Input: dimensioned drawing with shaded views. Units: mm. Origin: part minimum x, y, z. A direction names the side the tool comes from. Round coordinates to 2 decimals unless told otherwise and drop trailing zeros. Order: outer loops, then holes, each group sorted by start corner. A loop starts at its lowest first (then second) coordinate and runs counter-clockwise, first axis right, second up. Notation, with made-up numbers: M -25,43.5 L 30,43.5 A21 cw 30,63.5 Z; hole C 22.5,66.25 d6. An arc over 180 degrees is marked long. Use one line per item in the form item = value. Start each with the question number.
Q1. Section D-D (x = 43). Return the cut outline in (y, z).
Q2. Material intervals for probe 1 along Y at (x, z) = (40, 2.5); probe 2 along Z at (x, y) = (7, 20.5); probe 3 along X at (y, z) = (29.5, 37.5), sorted ascending.
Q3. Pull-direction query (Z, two-part tool) for the marked faces 3, 4 and 5; classes: pulls with the +Z half, pulls with the -Z half, needs draft (parallel to the pull), parting line crosses it, or undercut.
Q4. Contact query for flat-ended pins moving along their axis: pin 1 (1.5 mm diameter, centred on y = 18, z = 12.5, fed in from -X); pin 2 (5 mm diameter, centred on x = 14, y = 3.5, fed in from +Z); pin 3 (16 mm diameter, centred on y = 21, z = 30, fed in from +X); pin 4 (20 mm diameter, centred on x = 31, y = 12, fed in from +Z). Output: stop coordinate, or through.
Q5. Section B-B (x = 7.5). Return the cut outline in (y, z).
Q6. Section A-A (z = 28). Return the cut outline in (x, y).
Q7. Section C-C (y = 29). Return the cut outline in (x, z), plus the area to 3 significant figures.
Q8. Reachability of the marked faces 1 and 2 from +Z, -Z, +X, -X, +Y, -Y: full face, straight path, thin tool, end or side. Return the list, or none.
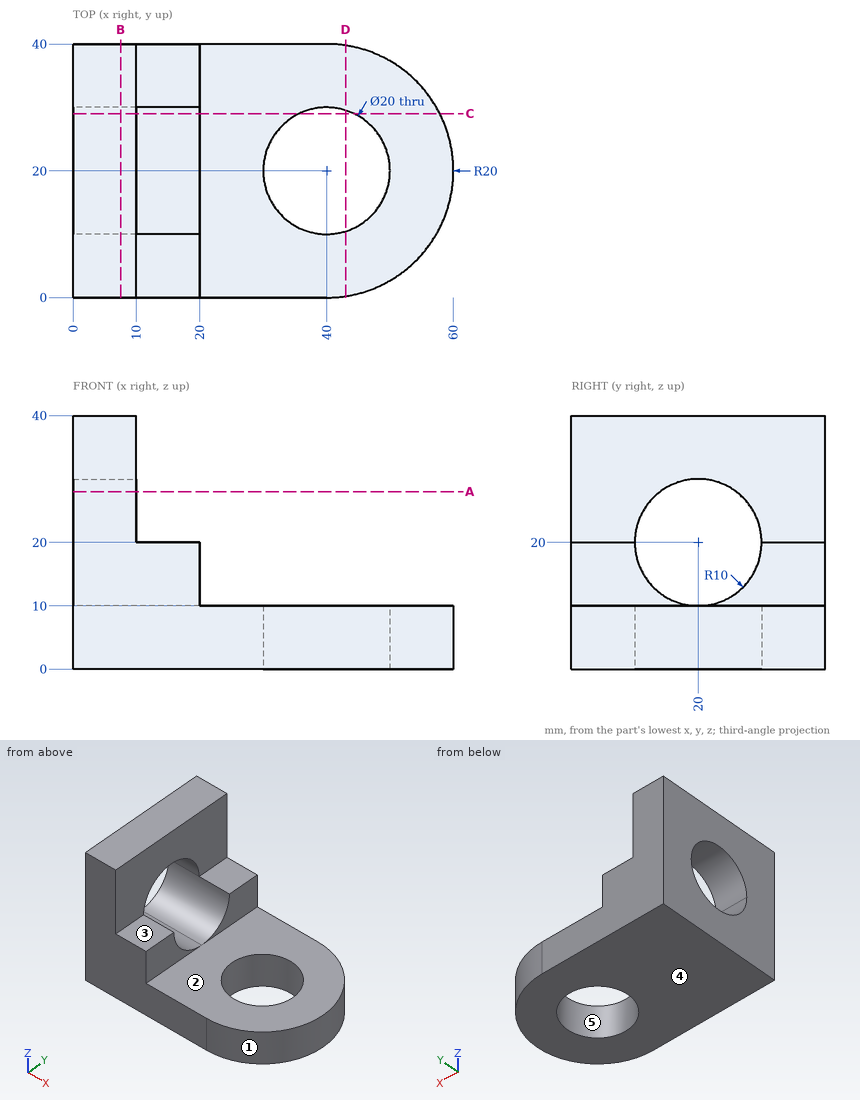
Results list:
q1.outline = M 0.23,0 L 10.46,0 L 10.46,10 L 0.23,10 Z; M 29.54,0 L 39.77,0 L 39.77,10 L 29.54,10 Z
q2.probe_1 = 0 to 10, 30 to 40
q2.probe_2 = 0 to 10.01, 29.99 to 40
q2.probe_3 = 0 to 10
q3.face_3 = pulls with the +Z half
q3.face_4 = pulls with the -Z half
q3.face_5 = needs draft
q4.pin_1 = through
q4.pin_2 = 20
q4.pin_3 = 10
q4.pin_4 = 10
q5.outline = M 0,0 L 40,0 L 40,40 L 0,40 Z; hole C 20,20 d20
q6.outline = M 0,0 L 10,0 L 10,14 L 0,14 Z; M 0,26 L 10,26 L 10,40 L 0,40 Z
q7.outline = M 0,0 L 35.64,0 L 35.64,10 L 20,10 L 20,15.64 L 0,15.64 Z; M 0,24.36 L 10,24.36 L 10,40 L 0,40 Z; M 44.36,0 L 57.86,0 L 57.86,10 L 44.36,10 Z
q7.area = 761 mm2
q8.face_1 = +Z, -Z, +X
q8.face_2 = +Z, +X, +Y, -Y
